Solid Edge part; units mm, degrees
sketch "Sketch1" plane through (0, 0, 0) normal (0, -1, 0) x (1, 0, 0)
  line L0 (45, 28) -> (10, 28)
  line L1 (10, 28) -> (10, 10)
  line L2 (0, 10) -> (10, 10)
  line L3 (0, 0) -> (0, 10)
  line L4 (0, 0) -> (0, -45)
  line L5 (0, -45) -> (50, -45)
  line L6 (50, -45) -> (50, 0)
  line L7 (50, 0) -> (50, 3)
  line L8 (50, 3) -> (45, 3)
  line L9 (45, 3) -> (45, 28)
extrude "Protrusion1" add sketch "Sketch1" along normal mid plane 100
hole "Hole_1" at (50, 0, -27) direction (-1, 0, 0) diameter 16 end through all
sketch "Sketch2" plane through (50, 0, -21) normal (1, 0, 0) x (0, 1, 0)
  line L0 (-20, -24) -> (-20, 21)
  line L1 (-20, 21) -> (-50, 21)
  line L2 (-50, 21) -> (-50, -24)
  line L3 (-50, -24) -> (-20, -24)
  line L4 (20, 21) -> (20, -24)
  line L5 (20, -24) -> (50, -24)
  line L6 (50, -24) -> (50, 21)
  line L7 (50, 21) -> (20, 21)
extrude "Cutout1" cut sketch "Sketch2" against normal through all
fillet "Round_1" radius 3 1 edges at (10, 0, 10)
fillet "Round_2" radius 10 1 edges at (10, 0, 28)
hole "Hole_2" at (45, -30, 15.5) direction (-1, 0, 0) diameter 4.134 depth 13 tip angle 118 thread major 5 thread length 10
hole "Hole1" at (45, 30, 16.2931) direction (-1, 0, 0) diameter 4.134 depth 13 tip angle 118 thread major 5 thread length 10
hole "Hole_4" at (25, 12, -45) direction (0, 0, 1) diameter 4.134 depth 13 thread major 5 thread length 10
hole "Hole2" at (25, -12, -45) direction (0, 0, 1) diameter 4.134 depth 13 thread major 5 thread length 10
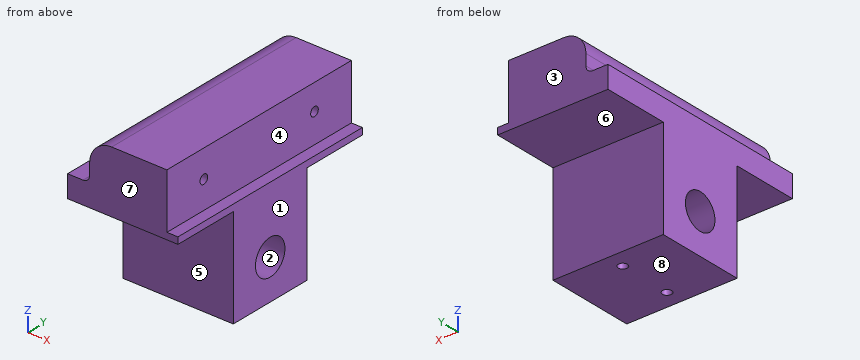
For this review, take the finished solid that the model builds, in its own axes (mm). Face numbers are marked on the shaded views. A direction names the side the tool comes from. Round coordinates to 2 decimals unless told otherwise and drop trailing zeros. Loops run counter-clockwise (first coordinate to the right, second up) from the corner with the lowest first, then second, coordinate; pieces in that order, holes last. Notation, with made-up numbers: (37.25, 24.5) - (44.25, 24.5) arc R8 ccw to (44.25, 30.5) - close; hole circle Ø3 at (71, -21). An arc over 180 degrees is marked (long way). Put each result on its own line as item: value. Start each with the question number.
1. Mouldability with a two-part tool opening along Y and no side actions: class the marked faces 1, 2 and 3 as +Y half, -Y half, draft (parallel to the pull), parting line (faces both ways), or undercut.
2. Consider section B-B on y = 0. State the section outline as (x, z) points.
3. For the marked faces 4, 5, 6, 7 and 8, list the 3-axis set-ups (+Z, -Z, +X, -X, +Y, -Y) from which the entire face can be reached by the end or side of a thin tool; tool diameter is ignored.
4. For probe 1 along Y at (x, z) = (25, -38); probe 2 along Y at (x, z) = (37.75, 15.5); probe 3 along Z at (x, y) = (42, -30), list the stretches that pass through material, from the lowest coordinate up. Write a range as [from, to].
5. Insertion check: P1, Ø7.5, axis at x = 2, y = -23, coming from the +Z side; P2, Ø1.5, axis at x = 11.5, z = -34, coming from the -Y side; P3, Ø10, axis at x = 37.5, y = 33.5, coming from the -Z side. Each pin has a flat end and moves straight along its axis. Give the tip position at first contact, or say it passes through.
6. Consider section C-C on x = 25. State the section outline as (y, z) points, plus the area to 3 significant figures.
7. Consider section A-A on z = -27. State the section outline as (x, y) points.
8. Consider section D-D on y = 12. State the section outline as (x, z) points, plus the area to 3 significant figures.
Result sheet:
1. face 1: draft
1. face 2: undercut
1. face 3: +Y half
2. outline: (0, -45) - (50, -45) - (50, -35) - (0, -35) - close; (0, -19) - (50, -19) - (50, 3) - (45, 3) - (45, 28) - (20, 28) arc R10 ccw to (10, 18) - (10, 13) arc R3 cw to (7, 10) - (0, 10) - close
3. face 4: +Z, +X, +Y, -Y
3. face 5: -Z, +X, -X, -Y
3. face 6: -Z, +X, -X, +Y
3. face 7: +Z, -Z, +X, -X, -Y
3. face 8: -Z, +X, -X, +Y, -Y
4. probe 1: [-20, -14.07], [-9.93, 9.93], [14.07, 20]
4. probe 2: [-50, -32.07], [-27.93, 28.09], [31.91, 50]
4. probe 3: [0, 13.43], [17.57, 28]
5. P1: z = 10
5. P2: y = -20
5. P3: z = 0
6. outline: (-50, 0) - (-20, 0) - (-20, -45) - (-14.07, -45) - (-14.07, -32) - (-9.93, -32) - (-9.93, -45) - (9.93, -45) - (9.93, -32) - (14.07, -32) - (14.07, -45) - (20, -45) - (20, 0) - (50, 0) - (50, 28) - (-50, 28) - close; hole circle Ø16 at (0, -27)
6. area: 4,290 mm^2
7. outline: (0, -20) - (50, -20) - (50, -8) - (0, -8) - close; (0, 8) - (50, 8) - (50, 20) - (0, 20) - close
8. outline: (0, -45) - (22.93, -45) - (22.93, -32) - (27.07, -32) - (27.07, -45) - (50, -45) - (50, 3) - (45, 3) - (45, 28) - (20, 28) arc R10 ccw to (10, 18) - (10, 13) arc R3 cw to (7, 10) - (0, 10) - close
8. area: 3,270 mm^2
